Build history of the part. All positions in model axes, mm. Round coordinates to 2 decimals unless told otherwise and drop trailing zeros. Write each loop counter-clockwise with the first axis right and the second up, starting at its lowest first coordinate (ties: lowest second). Pieces come first, ordered by that corner, then holes. Notation, with made-up numbers: M -30,-38.5 L -8,-38.5 A22 cw -8,0.5 Z; hole C -10,40.5 d1. An arc over 180 degrees is marked long. Write item = value, one per line.
from build123d import *

# Parameters (mm, degrees)
SKETCH_1_W          = 34
SKETCH_1_H          = 8
SKETCH_1_R          = 1.5
EXTRUDE_1_DEPTH     = 8
SKETCH_2_R          = 1.5
CUT_EXTRUDE_1_DEPTH = 8
SKETCH_3_R          = 1.5
CUT_EXTRUDE_2_DEPTH = 39


with BuildPart() as part:
    # 草图1 → 凸台-拉伸1 (new body)
    with BuildSketch(Plane(origin=(0, 0, 0), x_dir=(1, 0, 0), z_dir=(0, 1, 0))):
        Rectangle(SKETCH_1_W, SKETCH_1_H)
        with Locations(Location((-9, 0, 0), (0, 0, 270))):
            Circle(SKETCH_1_R, mode=Mode.SUBTRACT)
        with Locations(Location((9, 0, 0), (0, 0, 270))):
            Circle(SKETCH_1_R, mode=Mode.SUBTRACT)
    extrude(amount=EXTRUDE_1_DEPTH)

    # 草图2 → 切除-拉伸1 (cut)
    with BuildSketch(Plane.XY.offset(4)):
        with Locations((-4, 4)):
            Circle(SKETCH_2_R)
        with Locations(Location((4, 4, 0), (0, 0, 180))):
            Circle(SKETCH_2_R)
    extrude(amount=-CUT_EXTRUDE_1_DEPTH, mode=Mode.SUBTRACT)

    # 草图3 → 切除-拉伸2 (cut)
    with BuildSketch(Plane.ZY.offset(17)):
        with Locations((0, 4)):
            Circle(SKETCH_3_R)
    extrude(amount=-CUT_EXTRUDE_2_DEPTH, mode=Mode.SUBTRACT)


solid = part.part
1. Band-saw the part on A-A (z = -3). List the corners of the cut face in (x, y), plus the area to 3 significant figures.
Responses:
outline = M -17,0 L 17,0 L 17,8 L -17,8 Z; hole C -4,4 d3; hole C 4,4 d3
area = 258 mm²
2. Band-saw the part on B-B (x = 8.5). List the corners of the cut face in (y, z), plus the area to 3 significant figures.
Responses:
outline = M 0,-4 L 8,-4 L 8,-1.41 L 4.5,-1.41 A1.5 cw 3.5,-1.41 L 0,-1.41 Z; M 0,1.41 L 3.5,1.41 A1.5 cw 4.5,1.41 L 8,1.41 L 8,4 L 0,4 Z
area = 41.3 mm²
3. Band-saw the part on D-D (y = 3.5). Count the separate pieces of the cut face and the enclosed holes in it, plus the area to 3 significant figures.
Responses:
separate_pieces = 6
enclosed_holes = 0
area = 146 mm²
4. Flat gauge pins, fed straight in: pin 1 (4 mm diameter, centred on x = -4, y = 4, fed in from +Z); pin 2 (2.5 mm diameter, centred on x = 4, y = 4, fed in from +Z). Where does each tip first touch, or does it go through?
Responses:
pin_1 = 4
pin_2 = through
5. Probe probe 1 along Z at (x, y) = (-15, 4); probe 2 along Y at (x, z) = (-4, 1.8); probe 3 along X at (y, z) = (2, 0.25). List the from-to ranges inside material, lowest first.
Responses:
probe_1 = -4 to -1.5, 1.5 to 4
probe_2 = 0 to 2.5, 5.5 to 8
probe_3 = -17 to -10.48, -7.52 to 7.52, 10.48 to 17
6. Mould opens along Z. For faces 1 (the face through (9.07, 6.42, -1.5)), 2 (the face through (-2.57, 4.45, -2.42)), 3 (the face through (0, 4, -4)) say: pulls with the +Z half, pulls with the -Z half, needs draft (parallel to the pull), parting line crosses it, or undercut.
Responses:
face_1 = undercut
face_2 = needs draft
face_3 = pulls with the -Z half
7. Band-saw the part on C-C (y = 1.75). List the corners of the cut face in (x, z), plus the area to 3 significant figures.
Responses:
outline = M -17,-4 L 17,-4 L 17,4 L -17,4 Z; hole C -9,0 d3; hole C 9,0 d3
area = 258 mm²
